from build123d import *

# Parameters (mm, degrees)
SKETCH1_W                = 42.2
SKETCH1_H                = 42.2
SKETCH1_W_2              = 23.5
SKETCH1_H_2              = 23.5
BOSS_EXTRUDE1_DEPTH      = 5
SKETCH3_W                = 11.5
SKETCH3_H                = 3
BOSS_EXTRUDE3_DEPTH      = 1.5
CHAMFER1_SIZE            = 3.8
FILLET1_R                = 3
FILLET2_R                = 1
CHAMFER3_SIZE            = 0.5
CHAMFER4_SIZE            = 0.6
BOSS_EXTRUDE5_DEPTH      = 5
BOSS_EXTRUDE5_DEPTH_BACK = 10
CHAMFER5_SIZE            = 0.4
CUT_EXTRUDE4_START       = -10
SKETCH8_W                = 22
SKETCH8_H                = 2.5
CUT_EXTRUDE4_DEPTH       = 10
CHAMFER6_SIZE            = 1


with BuildPart() as part:
    # Sketch1 → Boss-Extrude1 (new body)
    with BuildSketch(Plane.XY):
        Rectangle(SKETCH1_W, SKETCH1_H)
        Rectangle(SKETCH1_W_2, SKETCH1_H_2, mode=Mode.SUBTRACT)
    extrude(amount=BOSS_EXTRUDE1_DEPTH)

    # Sketch3 → Boss-Extrude3 (add)
    with BuildSketch(Plane.XY.offset(5)):
        Polygon((11.75, 11.75), (5.75, 11.75), (5.75, 8.75), (5.75, 5), (-5.75, 5), (-5.75, 8.75), (-5.75, 11.75), (-11.75, 11.75), (-11.75, -11.75), (-5.75, -11.75), (-5.75, -8.75), (-5.75, -5), (5.75, -5), (5.75, -8.75), (5.75, -11.75), (11.75, -11.75), align=None)
        with Locations((0, 10.25)):
            Rectangle(SKETCH3_W, SKETCH3_H)
        with Locations((0, -10.25)):
            Rectangle(SKETCH3_W, SKETCH3_H)
    extrude(amount=-BOSS_EXTRUDE3_DEPTH)

    # Chamfer1
    chamfer1_edges = [part.edges().sort_by_distance(p)[0] for p in [
        (21.1, -21.1, 2.5),
        (-21.1, -21.1, 2.5),
        (-21.1, 21.1, 2.5),
        (21.1, 21.1, 2.5),
    ]]
    chamfer(chamfer1_edges, length=CHAMFER1_SIZE)

    # Fillet1
    fillet1_edges = [part.edges().sort_by_distance(p)[0] for p in [
        (-11.75, -11.75, 1.75),
        (11.75, -11.75, 1.75),
        (-11.75, 11.75, 1.75),
        (11.75, 11.75, 1.75),
    ]]
    fillet(fillet1_edges, radius=FILLET1_R)

    # Fillet2
    fillet2_edges = [part.edges().sort_by_distance(p)[0] for p in [
        (5.75, 8.75, 4.25),
        (-5.75, 8.75, 4.25),
        (-5.75, 5, 4.25),
        (5.75, -8.75, 4.25),
        (5.75, -5, 4.25),
        (-5.75, -5, 4.25),
        (5.75, 5, 4.25),
        (-5.75, -8.75, 4.25),
    ]]
    fillet(fillet2_edges, radius=FILLET2_R)

    # Chamfer3
    chamfer3_edges = [part.edges().sort_by_distance(p)[0] for p in [
        (-10.871320344, -10.871320344, 0),
        (-10.871320344, 10.871320344, 0),
        (10.871320344, -10.871320344, 0),
        (10.871320344, 10.871320344, 0),
        (-11.75, 0, 0),
        (0, -11.75, 0),
        (0, 11.75, 0),
        (11.75, 0, 0),
    ]]
    chamfer(chamfer3_edges, length=CHAMFER3_SIZE)

    # Chamfer4
    chamfer4_edges = [part.edges().sort_by_distance(p)[0] for p in [
        (0, -8.75, 5),
        (-5.75, -6.875, 5),
        (0, -5, 5),
        (5.75, -6.875, 5),
        (5.75, 6.875, 5),
        (0, 5, 5),
        (-5.75, 6.875, 5),
        (0, 8.75, 5),
        (-5.457106781, -8.457106781, 5),
        (-5.457106781, -5.292893219, 5),
        (5.457106781, -5.292893219, 5),
        (5.457106781, -8.457106781, 5),
        (5.457106781, 5.292893219, 5),
        (-5.457106781, 5.292893219, 5),
        (-5.457106781, 8.457106781, 5),
        (5.457106781, 8.457106781, 5),
        (0, 21.1, 5),
        (21.1, 0, 5),
        (-21.1, 0, 5),
        (0, -21.1, 5),
        (-19.2, -19.2, 5),
        (-19.2, 19.2, 5),
        (19.2, -19.2, 5),
        (19.2, 19.2, 5),
    ]]
    chamfer(chamfer4_edges, length=CHAMFER4_SIZE)

    # Sketch7 → Boss-Extrude5 (add, two sides)
    with BuildSketch(Plane.XY) as boss_extrude5_sk:
        Polygon((18.335533906, 23.6), (-18.335533906, 23.6), (-23.6, 18.335533906), (-23.6, -18.335533906), (-18.335533906, -23.6), (18.335533906, -23.6), (23.6, -18.335533906), (23.6, 18.335533906), align=None)
        Polygon((17.3, 21.1), (-17.3, 21.1), (-21.1, 17.3), (-21.1, -17.3), (-17.3, -21.1), (17.3, -21.1), (21.1, -17.3), (21.1, 17.3), align=None, mode=Mode.SUBTRACT)
    extrude(amount=BOSS_EXTRUDE5_DEPTH)
    extrude(boss_extrude5_sk.sketch, amount=-BOSS_EXTRUDE5_DEPTH_BACK)

    # Chamfer5
    chamfer5_edges = [part.edges().sort_by_distance(p)[0] for p in [
        (20.967766953, 20.967766953, 5),
        (0, 23.6, 5),
        (-20.967766953, 20.967766953, 5),
        (-23.6, 0, 5),
        (-20.967766953, -20.967766953, 5),
        (0, -23.6, 5),
        (20.967766953, -20.967766953, 5),
        (23.6, 0, 5),
        (-19.2, 19.2, 5),
        (-21.1, 0, 5),
        (-19.2, -19.2, 5),
        (0, -21.1, 5),
        (19.2, -19.2, 5),
        (21.1, 0, 5),
        (19.2, 19.2, 5),
        (0, 21.1, 5),
    ]]
    chamfer(chamfer5_edges, length=CHAMFER5_SIZE)

    # Sketch8 → Cut-Extrude4 (cut)
    with BuildSketch(Plane(origin=(0, 0, -10), x_dir=(-1, 0, 0), z_dir=(0, 0, -1)).offset(CUT_EXTRUDE4_START)):
        with Locations((0, -22.35)):
            Rectangle(SKETCH8_W, SKETCH8_H)
    extrude(amount=CUT_EXTRUDE4_DEPTH, mode=Mode.SUBTRACT)

    # Chamfer6
    chamfer6_edges = [part.edges().sort_by_distance(p)[0] for p in [
        (20.967766953, 20.967766953, -10),
        (0, 23.6, -10),
        (-20.967766953, 20.967766953, -10),
        (-23.6, 0, -10),
        (-20.967766953, -20.967766953, -10),
        (-14.667766953, -23.6, -10),
        (20.967766953, -20.967766953, -10),
        (23.6, 0, -10),
        (14.667766953, -23.6, -10),
        (11, -22.35, -10),
        (-11, -22.35, -10),
    ]]
    chamfer(chamfer6_edges, length=CHAMFER6_SIZE)


solid = part.part
Model file for the job. Use its own axes, mm. A direction names the side the tool comes from. Round coordinates to 2 decimals unless told otherwise and drop trailing zeros. Order: outer loops, then holes, each group sorted by start corner. A loop starts at its lowest first (then second) coordinate and runs counter-clockwise, first axis right, second up.
(1) Drill centre lines: line 1 (X direction, y = 15.5, z = 4.75); line 2 (X direction, y = -12.5, z = -1.75); line 3 (Y direction, x = 7, z = 1). Where is each one in solid material? Low to high.
(2) Pin check, flat tips, straight feed: pin 1 (4 mm diameter, centred on x = -12, y = -6.5, fed in from -Z); pin 2 (2 mm diameter, centred on x = 5, y = -4, fed in from -Z); pin 3 (5 mm diameter, centred on x = 6.5, z = -6, fed in from -Y). Stop position of each tip, or through.
(3) Band-saw the part on D-D (x = 2). Give the number of separate pieces and of enclosed holes in the cut face, then the cut area to 3 significant figures.
(4) 3-axis set-ups, long thin cutter, end or side, ignore diameter. For faces 1 (the face through (-5.62, 5.12, 4.64)), 2 (the face through (-11.75, 0, 2)), 3 (the face through (-21.005, -20.931, -2.105)): which of +Z, -Z, +X, -X, +Y, -Y reach the whole face in a straight line?
(5) Band-saw the part on B-B (x = -15.5). List the corners of the cut face in (y, z).
Verdict:
1. line 1: x = -23.45 to -21.25, -20.75 to 20.75, 21.25 to 23.45
1. line 2: x = -23.6 to -21.1, 21.1 to 23.6
1. line 3: y = -23.6 to -11.75, 11.75 to 23.6
2. pin 1: stops at z = 0
2. pin 2: stops at z = 3.5
2. pin 3: stops at y = 21.1
3. separate pieces: 3
3. enclosed holes: 0
3. area: 165 mm2
4. face 1: +Z
4. face 2: -Z
4. face 3: +Z, -Z, -X, -Y
5. outline: (-23.6, -9) - (-22.6, -10) - (-21.1, -10) - (-21.1, 0) - (21.1, 0) - (21.1, -10) - (22.6, -10) - (23.6, -9) - (23.6, 4.6) - (23.2, 5) - (21.5, 5) - (21.1, 4.6) - (21.1, 4.4) - (20.5, 5) - (-20.5, 5) - (-21.1, 4.4) - (-21.1, 4.6) - (-21.5, 5) - (-23.2, 5) - (-23.6, 4.6) - close
